```python
from build123d import *
from build123d.topology import SkipClean

# Parameters (mm, degrees)
BOSS_EXTRUDE1_DEPTH = 4
BOSS_EXTRUDE2_DEPTH = 2.5
SKETCH3_R           = 7.925
CUT_EXTRUDE1_DEPTH  = 9.25
SKETCH4_R           = 2
CUT_EXTRUDE2_DEPTH  = 9.25
CUT_EXTRUDE3_DEPTH  = 3.25
FILLET1_R           = 2.36
CHAMFER1_SIZE       = 3.5
CHAMFER1_SIZE2      = 2.020725942
BOSS_EXTRUDE4_DEPTH = 4
FILLET4_R           = 2
BOSS_EXTRUDE5_START = 2.25
SKETCH11_R          = 11.925
BOSS_EXTRUDE5_DEPTH = 2.25
CUT_EXTRUDE4_START  = -2.25
SKETCH12_R          = 7.925
CUT_EXTRUDE4_DEPTH  = 2.25


with BuildPart() as part:
    # Sketch1 → Boss-Extrude1 (new body)
    with BuildSketch(Plane(origin=(0, 0, 0), x_dir=(1, 0, 0), z_dir=(0, 1, 0))):
        with BuildLine():
            Line((-13.29118379, 20.889836125), (-0.68999579, 20.889836125))
            Line((-0.68999579, 20.889836125), (-0.68999579, 26.09210312))
            Line((-0.68999579, 26.09210312), (12.01000421, 26.09210312))
            Line((12.01000421, 26.09210312), (12.01000421, -28.90789688))
            Line((12.01000421, -28.90789688), (-0.68999579, -28.90789688))
            Line((-0.68999579, -28.90789688), (-0.68999579, -23.705629885))
            Line((-0.68999579, -23.705629885), (-13.29118379, -23.705629885))
            ThreePointArc((-13.29118379, -23.705629885), (-35.588916795, -1.40789688), (-13.29118379, 20.889836125))
        make_face()
    extrude(amount=BOSS_EXTRUDE1_DEPTH)

    # Sketch2 → Boss-Extrude2 (add)
    with BuildSketch(Plane(origin=(0, 4, 0), x_dir=(1, 0, 0), z_dir=(0, 1, 0))):
        with BuildLine():
            Line((-13.29118379, 20.889836125), (-0.68999579, 20.889836125))
            Line((-0.68999579, 20.889836125), (-0.68999579, 16.987726462))
            ThreePointArc((-0.68999579, 16.987726462), (9.006549215, -1.40789688), (-0.68999579, -19.803520222))
            Line((-0.68999579, -19.803520222), (-0.68999579, -23.705629885))
            Line((-0.68999579, -23.705629885), (-13.29118379, -23.705629885))
            ThreePointArc((-13.29118379, -23.705629885), (-35.588916795, -1.40789688), (-13.29118379, 20.889836125))
        make_face()
    extrude(amount=BOSS_EXTRUDE2_DEPTH)

    # Sketch3 → Cut-Extrude1 (cut)
    with BuildSketch(Plane.XZ):
        with Locations(Location((-13.29118379, 1.40789688, 0), (0, 0, 270))):
            Circle(SKETCH3_R)
    extrude(amount=-CUT_EXTRUDE1_DEPTH, mode=Mode.SUBTRACT)

    # Sketch4 → Cut-Extrude2 (cut)
    with BuildSketch(Plane.XZ):
        with Locations(Location((3.31000421, 24.40789688, 0), (0, 0, 270))):
            Circle(SKETCH4_R)
        with Locations(Location((3.310004206, -21.59210312, 0), (0, 0, 270))):
            Circle(SKETCH4_R)
    extrude(amount=-CUT_EXTRUDE2_DEPTH, mode=Mode.SUBTRACT)

    # Sketch5 → Cut-Extrude3 (cut)
    with BuildSketch(Plane.XZ):
        with BuildLine():
            ThreePointArc((-20.901279021, -7.773174712), (-25.21618379, 1.40789688), (-20.901279021, 10.588968471))
            Line((-20.901279021, 10.588968471), (-24.18129969, 16.27013092))
            ThreePointArc((-24.18129969, 16.27013092), (-31.71618379, 1.40789688), (-24.18129969, -13.454337161))
            Line((-24.18129969, -13.454337161), (-20.901279021, -7.773174712))
        make_face()
        with BuildLine():
            Line((-20.717198075, 18.27013092), (-17.437177406, 12.588968471))
            ThreePointArc((-17.437177406, 12.588968471), (-7.32868379, 11.73524982), (-1.535094942, 3.40789688))
            Line((-1.535094942, 3.40789688), (5.024946397, 3.40789688))
            ThreePointArc((5.024946397, 3.40789688), (-4.07868379, 17.364414944), (-20.717198075, 18.27013092))
        make_face()
        with BuildLine():
            ThreePointArc((-1.535094942, -0.59210312), (-7.32868379, -8.91945606), (-17.437177406, -9.773174712))
            Line((-17.437177406, -9.773174712), (-20.717198075, -15.454337161))
            ThreePointArc((-20.717198075, -15.454337161), (-4.07868379, -14.548621185), (5.024946397, -0.59210312))
            Line((5.024946397, -0.59210312), (-1.535094942, -0.59210312))
        make_face()
    extrude(amount=-CUT_EXTRUDE3_DEPTH, mode=Mode.SUBTRACT)

    # Fillet1
    fillet1_edges = [part.edges().sort_by_distance(p)[0] for p in [
        (-20.901279021, 1.625, 10.588968471),
        (-20.901279021, 1.625, -7.773174712),
        (-24.18129969, 1.625, -13.454337161),
        (-24.18129969, 1.625, 16.27013092),
        (5.024946397, 1.625, 3.40789688),
        (-1.535094942, 1.625, 3.40789688),
        (-20.717198075, 1.625, 18.27013092),
        (-1.535094942, 1.625, -0.59210312),
        (5.024946397, 1.625, -0.59210312),
        (-20.717198075, 1.625, -15.454337161),
    ]]
    fillet(fillet1_edges, radius=FILLET1_R)

    # Chamfer1
    chamfer1_edges = [part.edges().sort_by_distance(p)[0] for p in [
        (12.01000421, 0, 1.40789688),
    ]]
    chamfer1_side = [part.faces().sort_by_distance(p)[0] for p in [
        (-3.714999267, 0, 17.994335016),
    ]]
    chamfer(chamfer1_edges, length=CHAMFER1_SIZE, length2=CHAMFER1_SIZE2, reference=chamfer1_side[0])

    # Sketch10 → Boss-Extrude4 (add)
    with BuildSketch(Plane.XZ):
        with BuildLine():
            Line((-0.68999579, -22.889836125), (-13.29118379, -22.889836125))
            ThreePointArc((-13.29118379, -22.889836125), (-37.588916795, 1.40789688), (-13.29118379, 25.705629885))
            Line((-13.29118379, 25.705629885), (-0.68999579, 25.705629885))
            Line((-0.68999579, 25.705629885), (-0.68999579, 23.705629885))
            Line((-0.68999579, 23.705629885), (-13.29118379, 23.705629885))
            ThreePointArc((-13.29118379, 23.705629885), (-35.588916795, 1.40789688), (-13.29118379, -20.889836125))
            Line((-13.29118379, -20.889836125), (-0.68999579, -20.889836125))
            Line((-0.68999579, -20.889836125), (-0.68999579, -22.889836125))
        make_face()
    extrude(amount=-BOSS_EXTRUDE4_DEPTH)

    # Fillet4
    fillet4_edges = [part.edges().sort_by_distance(p)[0] for p in [
        (-6.99058979, 0, 25.705629885),
        (-37.588916795, 0, 1.40789688),
        (-6.99058979, 0, -22.889836125),
    ]]
    fillet(fillet4_edges, radius=FILLET4_R)

    # Sketch11 → Boss-Extrude5 (add)
    with SkipClean():  # the faces are left unmerged after this step: merging them gives an invalid solid
        with BuildSketch(Plane.XZ.offset(BOSS_EXTRUDE5_START)):
            with Locations(Location((-13.29118379, 1.40789688, 0), (0, 0, 270))):
                Circle(SKETCH11_R)
        extrude(amount=-BOSS_EXTRUDE5_DEPTH)

    # Sketch12 → Cut-Extrude4 (cut)
    with SkipClean():  # the faces are left unmerged after this step: merging them gives an invalid solid
        with BuildSketch(Plane(origin=(0, 0, 0), x_dir=(1, 0, 0), z_dir=(0, 1, 0)).offset(CUT_EXTRUDE4_START)):
            with Locations(Location((-13.29118379, -1.40789688, 0), (0, 0, 270))):
                Circle(SKETCH12_R)
        extrude(amount=CUT_EXTRUDE4_DEPTH, mode=Mode.SUBTRACT)


solid = part.part
```
For this review, take the finished solid that the model builds, in its own axes (mm). A direction names the side the tool comes from. Round coordinates to 2 decimals unless told otherwise and drop trailing zeros. Write each loop counter-clockwise with the first axis right and the second up, starting at its lowest first coordinate (ties: lowest second). Pieces come first, ordered by that corner, then holes. Notation, with made-up numbers: (55, 16) -> (80, 16) arc R13 cw to (80, 27) -> close; hole circle Ø10 at (9.25, 67.5). An arc over 180 degrees is marked (long way). Use one line per item in the form item = value.
1) Tool access review of faces 4 (the flat face through (-18.351, 1.602, -11.355)), 5 (the cylindrical face through (-7.08, 0.57, -22.29)), 6 (the flat face through (6, 2, 28.908)): name each direction out of +Z, -Z, +X, -X, +Y, -Y from which nothing blocks a thin tool from reaching the whole face with its end or side.
Found:
face_4 = -Y
face_5 = -Z, -X, -Y
face_6 = +Z, +X, -X, +Y, -Y
2) Clearance check with flat-ended pins moving along their axes: pin 1 (1.2 mm diameter, centred on x = -6.5, y = 4.5, fed in from +Z); pin 2 (3 mm diameter, centred on x = -22, y = 5, fed in from +Z); pin 3 (10 mm diameter, centred on x = -31.5, z = 6.5, fed in from -Y). State where each tip first meets the part, or that it passes through.
Found:
pin_1 = 25.71
pin_2 = 24.49
pin_3 = 0
3) Mouldability with a two-part tool opening along X and no side actions: class faces 1 (the flat face through (-7, 5, -20.89)), 2 (the cylindrical face through (-35.584, 5.232, 1.898)), 3 (the cylindrical face through (-1.096, 1.648, 3.874)) as +X half, -X half, draft (parallel to the pull), parting line (faces both ways), or undercut.
Found:
face_1 = draft
face_2 = -X half
face_3 = undercut
4) To check wall thickness, follow L1, parallel to X at y = 0.75, z = -1; L2, parallel to Z at x = -16, y = 3; L3, parallel to Z at x = -17, y = 1.25. State the ranges of each line that lie inside material, in increasing order. Write a range as from..to.
Found:
L1 = -37.03..-31.56, -24.97..-20.84, -5.74..-1.01, 3.5..9.81
L2 = -22.74..-16.82, -10.21..-6.04, 8.86..13.02, 19.63..25.55
L3 = -22.46..-16.64, -9.93..-5.6, 8.41..12.74, 19.46..25.27
5) Take a section at A-A, the plane y = 5. Write out the cut boundary in (x, z) (3 decimals), and give its area (3 significant figures).
Found:
outline = (-13.291, -20.89) -> (-0.69, -20.89) -> (-0.69, -16.988) arc R22.298 ccw to (-0.69, 19.804) -> (-0.69, 23.706) -> (-13.291, 23.706) arc R22.298 ccw to start; hole circle Ø15.85 at (-13.291, 1.408)
area = 1,400 mm2
6) Take a section at B-B, the plane y = 0.75. Count the separate pieces of the cut face and the enclosed holes in it, and give its area (3 significant figures).
Found:
separate_pieces = 1
enclosed_holes = 6
area = 1,320 mm2
